```python
from build123d import *

# Parameters (mm, degrees)
SKETCH_1_W          = 160
SKETCH_1_H          = 55
EXTRUDE_1_DEPTH     = 5
SKETCH_2_R          = 3.5
SKETCH_2_W          = 9
SKETCH_2_H          = 11
SKETCH_2_W_2        = 12
SKETCH_2_H_2        = 18
SKETCH_2_W_3        = 2.5
SKETCH_2_H_3        = 10.5
CUT_EXTRUDE_1_DEPTH = 5
SKETCH_3_R          = 1.5
CUT_EXTRUDE_2_DEPTH = 10
FILLET_1_R          = 5
SKETCH_5_W          = 160
SKETCH_5_H          = 55
EXTRUDE_2_DEPTH     = 10
SKETCH_6_W          = 150
SKETCH_6_H          = 45
CUT_EXTRUDE_3_DEPTH = 10
SKETCH_3_2_R        = 1.5
CUT_EXTRUDE_4_DEPTH = 86.914201512


with BuildPart() as part:
    # Эскиз1 → Бобышка-Вытянуть1 (new body)
    with BuildSketch(Plane.XY):
        Rectangle(SKETCH_1_W, SKETCH_1_H)
    extrude(amount=EXTRUDE_1_DEPTH)

    # Эскиз2 → Вырез-Вытянуть1 (cut)
    with BuildSketch(Plane.XY.offset(5)):
        with Locations((60, -7.5)):
            Circle(SKETCH_2_R)
        with Locations((47, -7.5)):
            Rectangle(SKETCH_2_W, SKETCH_2_H)
        with Locations((30, -7.5)):
            Rectangle(SKETCH_2_W_2, SKETCH_2_H_2)
        with Locations((20, -7.5)):
            Rectangle(SKETCH_2_W_3, SKETCH_2_H_3)
    extrude(amount=-CUT_EXTRUDE_1_DEPTH, mode=Mode.SUBTRACT)

    # Эскиз3 → Вырез-Вытянуть2 (cut)
    with BuildSketch(Plane.XY.offset(5)):
        with Locations((-75, 22.5)):
            Circle(SKETCH_3_R)
        with Locations((-75, -22.5)):
            Circle(SKETCH_3_R)
        with Locations((75, 22.5)):
            Circle(SKETCH_3_R)
        with Locations((75, -22.5)):
            Circle(SKETCH_3_R)
    extrude(amount=-CUT_EXTRUDE_2_DEPTH, mode=Mode.SUBTRACT)

    # Скругление1
    # the kernel refuses this fillet: 5 mm, written as the material it takes off along each edge
    with BuildSketch(Plane(origin=(-80, 40, 5), x_dir=(0, 0, -1), z_dir=(0, -1, 0)), Plane(origin=(80, -40, 5), x_dir=(0, 0, -1), z_dir=(0, 1, 0))) as fillet_1_piece_1:
        with BuildLine():
            CenterArc((FILLET_1_R, FILLET_1_R), FILLET_1_R, 180, 90)
            Line((0, FILLET_1_R), (0, 0))
            Line((0, 0), (FILLET_1_R, 0))
        make_face()
    extrude(amount=80, mode=Mode.SUBTRACT)
    with BuildSketch(Plane(origin=(92.5, 27.5, 5), x_dir=(0, -1, 0), z_dir=(-1, 0, 0))) as fillet_1_piece_2:
        with BuildLine():
            CenterArc((FILLET_1_R, -FILLET_1_R), FILLET_1_R, 90, 90)
            Line((0, -FILLET_1_R), (0, 0))
            Line((0, 0), (FILLET_1_R, 0))
        make_face()
    extrude(amount=185, mode=Mode.SUBTRACT)

    # Эскиз5 → Бобышка-Вытянуть2 (add)
    with BuildSketch(Plane(origin=(0, 0, 0), x_dir=(-1, 0, 0), z_dir=(0, 0, -1))):
        Rectangle(SKETCH_5_W, SKETCH_5_H)
    extrude(amount=EXTRUDE_2_DEPTH)

    # Эскиз6 → Вырез-Вытянуть3 (cut)
    with BuildSketch(Plane(origin=(0, 0, -10), x_dir=(-1, 0, 0), z_dir=(0, 0, -1))):
        Rectangle(SKETCH_6_W, SKETCH_6_H)
    extrude(amount=-CUT_EXTRUDE_3_DEPTH, mode=Mode.SUBTRACT)

    # Эскиз3<2> → Вырез-Вытянуть4 (cut, through all)
    with BuildSketch(Plane.XY.offset(5)):
        with Locations((-75, 22.5)):
            Circle(SKETCH_3_2_R)
        with Locations(Location((-75, -22.5, 0), (0, 0, 90))):
            Circle(SKETCH_3_2_R)
        with Locations(Location((75, 22.5, 0), (0, 0, 270))):
            Circle(SKETCH_3_2_R)
        with Locations(Location((75, -22.5, 0), (0, 0, 90))):
            Circle(SKETCH_3_2_R)
    extrude(amount=-CUT_EXTRUDE_4_DEPTH, mode=Mode.SUBTRACT)


solid = part.part
```
For this review, take the finished solid that the model builds, in its own axes (mm). A direction names the side the tool comes from. Round coordinates to 2 decimals unless told otherwise and drop trailing zeros. Write each loop counter-clockwise with the first axis right and the second up, starting at its lowest first coordinate (ties: lowest second). Pieces come first, ordered by that corner, then holes.
1) Take a section at A-A on z = -7.5. Give the boundary of the cut face in (x, y), then the cut area to 3 significant figures.
Answer below:
outline: (-80, -27.5) - (80, -27.5) - (80, 27.5) - (-80, 27.5) - close; hole (-75, -21) arc R1.5 ccw (long way) to (-73.5, -22.5) - (73.5, -22.5) arc R1.5 ccw (long way) to (75, -21) - (75, 21) arc R1.5 ccw (long way) to (73.5, 22.5) - (-73.5, 22.5) arc R1.5 ccw (long way) to (-75, 21) - close
area: 2,030 mm2
2) Take a section at B-B on x = 44.5. Give the boundary of the cut face in (y, z).
Answer below:
outline: (-27.5, -10) - (-22.5, -10) - (-22.5, 0) - (-13, 0) - (-13, 5) - (-27.5, 5) - close; (-2, 0) - (22.5, 0) - (22.5, -10) - (27.5, -10) - (27.5, 0) arc R5 ccw to (22.5, 5) - (-2, 5) - close
3) Mouldability with a two-part tool opening along Y and no side actions: class faces 4 (the face through (47, -13, 3)), 5 (the face through (-1, -2, 5)), 6 (the face through (18.75, -8, 3)), 7 (the face through (1, 27.5, -5)) as +Y half, -Y half, draft (parallel to the pull), parting line (faces both ways), or undercut.
Answer below:
face 4: undercut
face 5: draft
face 6: undercut
face 7: +Y half
4) Take a section at D-D on z = 3. State how many separate pieces and enclosed holes the cut face has, then the cut area to 3 significant figures.
Answer below:
separate pieces: 1
enclosed holes: 8
area: 8,120 mm2
5) For line 1 along X through (y, z) = (-4, -0.75); line 2 along Y through (x, z) = (-29, -6.5); line 3 along Z through (x, y) = (-12.5, 0), list the stretches that pass through material, from the lowest coordinate up.
Answer below:
line 1: x = -80 to -75, 75 to 80
line 2: y = -27.5 to -22.5, 22.5 to 27.5
line 3: z = 0 to 5
6) Machinability: for faces 1 (the face through (-6, 23, -10)), 2 (the face through (36, -8, 3)), 3 (the face through (1, 22.5, -5)), which of the approach directions +Z, -Z, +X, -X, +Y, -Y give a long, thin tool a straight path to every point of the face, cutting with its end or side? Answer none if there is none.
Answer below:
face 1: -Z, +X, -X, +Y, -Y
face 2: +Z, -Z
face 3: -Z
7) Take a section at C-C on y = -7.5. Give the boundary of the cut face in (x, z).
Answer below:
outline: (-80, -10) - (-75, -10) - (-75, 0) - (18.75, 0) - (18.75, 5) - (-75, 5) arc R5 ccw to (-80, 0) - close; (21.25, 0) - (24, 0) - (24, 5) - (21.25, 5) - close; (36, 0) - (42.5, 0) - (42.5, 5) - (36, 5) - close; (51.5, 0) - (56.5, 0) - (56.5, 5) - (51.5, 5) - close; (63.5, 0) - (75, 0) - (75, -10) - (80, -10) - (80, 0) arc R5 ccw to (75, 5) - (63.5, 5) - close
8) Insertion check: pin 1 Ø2 at (x, y) = (47, 10.5) entering from -Z; pin 2 Ø5.5 at (y, z) = (-9.5, 3) entering from +X; pin 3 Ø5.5 at (y, z) = (-8, 3.5) entering from +X. Each pin has a flat end and moves straight along its axis. Give the tip position at first contact, or say it passes through.
Answer below:
pin 1: stops at z = 0
pin 2: stops at x = 79.99
pin 3: stops at x = 79.94
